For this review, take the finished solid that the model builds, in its own axes (mm). Face numbers are marked on the shaded views. Give positions to 0.01 mm unless a question says otherwise; leave off trailing zeros. Order: outer loops, then holes, each group sorted by start corner. A loop starts at its lowest first (then second) coordinate and runs counter-clockwise, first axis right, second up. Notation, with made-up numbers: (-7.5, 7.5) -> (30.5, 7.5) arc R32 cw to (30.5, 39.5) -> close; hole circle Ø3 at (35, -6.5). An arc over 180 degrees is marked (long way). Return JSON: item names as keys, results as strings. Group by question number.
1) The part is to be moulded in two halves that separate along Y. For the marked faces 1, 2 and 3, say which applies: released by +Y, released by -Y, zero draft, split by the parting line, or undercut.
2) Add section A-A (x = 0). Give the boundary of the cut face in (y, z).
3) To check wall thickness, follow line 1 along Y through (x, z) = (0, 5); line 2 along Z through (x, y) = (-11, -28); line 3 along Y through (x, z) = (1.5, 6) (3 decimals). State the ranges of each line that lie inside material, in increasing order.
4) Insertion check: P1, Ø10, axis at x = -51.5, z = 15, coming from the +Y side; P2, Ø1, axis at x = -44, y = -35, coming from the +Z side; P3, Ø10, axis at x = -50.37, z = 24.5, coming from the -Y side; P4, Ø1.5, axis at y = 30.5, z = 9, coming from the -X side. Each pin has a flat end and moves straight along its axis. Give the tip position at first contact, or say it passes through.
5) Add section C-C (z = 19). Give the boundary of the cut face in (x, y).
6) Add section D-D (x = 26.5). Give the boundary of the cut face in (y, z), then the cut area to 3 significant figures.
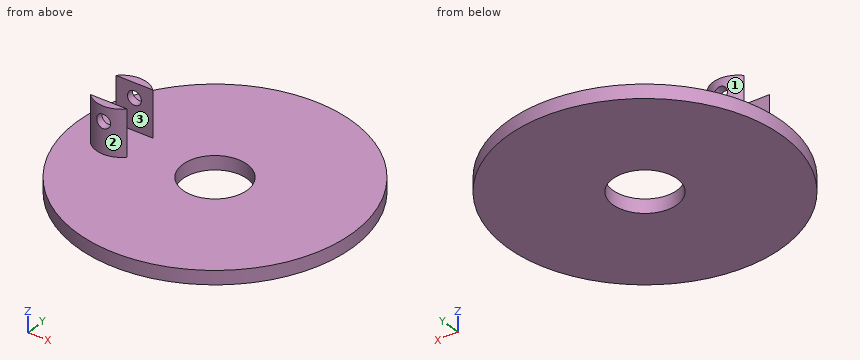
from build123d import *

# Parameters (mm, degrees)
SKETCH1_R               = 75
SKETCH1_R_2             = 17.5
BOSS_EXTRUDE2_DEPTH     = 7.5
SKETCH2_R               = 13.75
BOSS_EXTRUDE3_DEPTH     = 25
SKETCH3_OUTSIDE_W       = 194.922
SKETCH3_OUTSIDE_H       = 194.922
CUT_EXTRUDE3_DEPTH      = 25
SKETCH6_R               = 3.75
CUT_EXTRUDE4_DEPTH      = 85.5
CUT_EXTRUDE4_DEPTH_BACK = 66.5


with BuildPart() as part:
    # Sketch1 → Boss-Extrude2 (new body)
    with BuildSketch(Plane.XY):
        Circle(SKETCH1_R)
        Circle(SKETCH1_R_2, mode=Mode.SUBTRACT)
    extrude(amount=BOSS_EXTRUDE2_DEPTH)

    # Sketch2 → Boss-Extrude3 (add)
    with BuildSketch(Plane.XY.offset(7.5)):
        with Locations((-50.374404357, 0)):
            Circle(SKETCH2_R)
    extrude(amount=BOSS_EXTRUDE3_DEPTH)

    # Sketch3 outside → Cut-Extrude3 (cut)
    with BuildSketch(Plane.XY.offset(32.5)):
        Rectangle(SKETCH3_OUTSIDE_W, SKETCH3_OUTSIDE_H)
        with BuildLine():
            Line((-60.314852033, 9.5), (-40.433956681, 9.5))
            ThreePointArc((-40.433956681, 9.5), (-50.374404357, 13.75), (-60.314852033, 9.5))
        make_face(mode=Mode.SUBTRACT)
        with BuildLine():
            Line((-60.314852033, -9.5), (-40.433956681, -9.5))
            ThreePointArc((-40.433956681, -9.5), (-50.374404357, -13.75), (-60.314852033, -9.5))
        make_face(mode=Mode.SUBTRACT)
    extrude(amount=-CUT_EXTRUDE3_DEPTH, mode=Mode.SUBTRACT)

    # Sketch6 → Cut-Extrude4 (cut, two sides)
    with BuildSketch(Plane(origin=(0, -9.5, 0), x_dir=(1, 0, 0), z_dir=(0, 1, 0))) as cut_extrude4_sk:
        with Locations((-50.374404357, -24.5)):
            Circle(SKETCH6_R)
    extrude(amount=CUT_EXTRUDE4_DEPTH, mode=Mode.SUBTRACT)
    extrude(cut_extrude4_sk.sketch, amount=-CUT_EXTRUDE4_DEPTH_BACK, mode=Mode.SUBTRACT)


solid = part.part
Evaluation:
{
 "1": {"face 1": "released by +Y", "face 2": "released by -Y", "face 3": "undercut"},
 "2": {"outline": "(-75, 0) -> (-17.5, 0) -> (-17.5, 7.5) -> (-75, 7.5) -> close; (17.5, 0) -> (75, 0) -> (75, 7.5) -> (17.5, 7.5) -> close"},
 "3": {"line 1": "-75 to -17.5, 17.5 to 75", "line 2": "0 to 7.5", "line 3": "-74.985 to -17.436, 17.436 to 74.985"},
 "4": {"P1": "y = 13.75", "P2": "z = 7.5", "P3": "y = -13.75", "P4": "through"},
 "5": {"outline": "(-60.31, -9.5) arc R13.75 ccw to (-40.43, -9.5) -> close; (-60.31, 9.5) -> (-40.43, 9.5) arc R13.75 ccw to start"},
 "6": {"outline": "(-70.16, 0) -> (70.16, 0) -> (70.16, 7.5) -> (-70.16, 7.5) -> close", "area": "1,050 mm^2"}
}
